Geometry check sheet. Reference: the model listing, model coordinates, mm. A direction names the side the tool comes from. Round coordinates to 2 decimals unless told otherwise and drop trailing zeros. Order: outer loops, then holes, each group sorted by start corner. A loop starts at its lowest first (then second) coordinate and runs counter-clockwise, first axis right, second up.
```python
from build123d import *

# Parameters (mm, degrees)
F0_R     = 41.275
F1_DEPTH = 3.175
F2_R     = 15.603275
F3_DEPTH = 25.4
F4_R     = 7.62
F5_DEPTH = 25.4
F6_R     = 3.175
F8_R     = 3.175
F9_DEPTH = 25.4


with BuildPart() as f1:
    # F0 (on Front) → F1 (new body)
    with BuildSketch(Plane.XZ):
        Circle(F0_R)
    extrude(amount=F1_DEPTH)

    # F2 (on Front) → F3 (join)
    with BuildSketch(Plane.XZ):
        Circle(F2_R)
    extrude(amount=F3_DEPTH)

    # F4 (on Front) → F5 (cut)
    with BuildSketch(Plane.XZ):
        Circle(F4_R)
    extrude(amount=F5_DEPTH, mode=Mode.SUBTRACT)

    # F6
    f6_edges = [f1.edges().sort_by_distance(p)[0] for p in [
        (-15.603275, -3.175, 0),
    ]]
    fillet(f6_edges, radius=F6_R)

    # F8 (on face) → F9 (cut)
    with BuildSketch(Plane.XZ.offset(3.175)):
        with Locations((34.925, 0)):
            Circle(F8_R)
    extrude(amount=-F9_DEPTH, mode=Mode.SUBTRACT)


solid = f1.part
```
(1) Sectioned sample at A-A, the plane x = 0. Record the cut outline in (y, z) (3 decimals).
Returned:
outline: (-25.4, -15.603) - (-6.35, -15.603) arc R3.175 cw to (-3.175, -18.778) - (-3.175, -41.275) - (0, -41.275) - (0, -7.62) - (-25.4, -7.62) - close; (-25.4, 7.62) - (0, 7.62) - (0, 41.275) - (-3.175, 41.275) - (-3.175, 18.778) arc R3.175 cw to (-6.35, 15.603) - (-25.4, 15.603) - close
(2) Sectioned sample at C-C, the plane y = -8.75. Record the cut outline in (x, z).
Returned:
outline: circle Ø31.21 at (0, 0); hole circle Ø15.24 at (0, 0)
(3) Sectioned sample at B-B, the plane z = 0. Record the cut outline in (x, y) (3 decimals), and give its area (3 significant figures).
Returned:
outline: (-41.275, -3.175) - (-18.778, -3.175) arc R3.175 cw to (-15.603, -6.35) - (-15.603, -25.4) - (-7.62, -25.4) - (-7.62, 0) - (-41.275, 0) - close; (7.62, -25.4) - (15.603, -25.4) - (15.603, -6.35) arc R3.175 cw to (18.778, -3.175) - (31.75, -3.175) - (31.75, 0) - (7.62, 0) - close; (38.1, -3.175) - (41.275, -3.175) - (41.275, 0) - (38.1, 0) - close
area: 553 mm2
(4) Material ranges on line 1 (X direction, y = -1.5, z = -2); line 2 (Y direction, x = -21, z = -4.5) (3 decimals); line 3 (Z direction, x = -4, y = -24), recorded low to high.
Returned:
line 1: x = -41.23 to -7.35, 7.35 to 32.46, 37.39 to 41.23
line 2: y = -3.175 to 0
line 3: z = -15.08 to -6.49, 6.49 to 15.08
(5) Depth check by flat-ended pin: P1, Ø1, axis at x = -13.5, y = -12.5, coming from the -Z side; P2, Ø5, axis at x = 27.5, y = -4, coming from the -Z side; P3, Ø10, axis at x = 34.925, z = 0, coming from the -Y side (3 decimals); P4, Ø12, axis at x = -31.5, y = -11, coming from the +Z side. Enter the tip coordinate at first touch or a pass-through.
Returned:
P1: stops at z = -8.63
P2: stops at z = -32.74
P3: stops at y = -3.175
P4: passes through
(6) Draft check along Z on faces 1 (the cylindrical face through (-8.948, -1.565, -40.293)), 2 (the flat face through (-1, 0, -9)), 3 (the cylindrical face through (37.953, -1.61, 0.954)). Enter one of: released by +Z, released by -Z, zero draft, split by the parting line, or undercut.
Returned:
face 1: split by the parting line
face 2: zero draft
face 3: undercut
(7) Set-up check for faces 4 (the flat face through (7, -25.4, 4)), 5 (the flat face through (-19, -3.175, 1)): record each of +Z, -Z, +X, -X, +Y, -Y from which the full face is reachable in a straight line by a thin tool's end or side.
Returned:
face 4: +Z, -Z, +X, -X, -Y
face 5: -Y
(8) Sectioned sample at D-D, the plane z = -31.5. Record the cut outline in (x, y) (3 decimals).
Returned:
outline: (-26.672, -3.175) - (26.672, -3.175) - (26.672, 0) - (-26.672, 0) - close
